Geometry check sheet. Reference: the model listing, model coordinates, mm. Face numbers are marked on the shaded views. A direction names the side the tool comes from. Round coordinates to 2 decimals unless told otherwise and drop trailing zeros. Order: outer loops, then holes, each group sorted by start corner. A loop starts at its lowest first (then second) coordinate and runs counter-clockwise, first axis right, second up.
(1) Cross-section at A-A on y = 0. Enter the section's corners in (x, z) (3 decimals), and give its area (3 significant figures).
(2) Thickness scan on L1, parallel to Z at x = 5, y = 0; L2, parallel to X at y = -6.5, z = 0.5; L3, parallel to X at y = 1.5, z = 3.75. Record the ranges inside material, lowest first.
(3) Gauge pin test, flat ends, axial feed: P1, Ø4, axis at x = 19, z = -4, coming from the +Y side; P2, Ø1.5, axis at x = 13, z = 1.5, coming from the -Y side; P3, Ø1, axis at x = 4, z = -4, coming from the +Y side. Record the tip position at first contact, or that the pin passes through.
(4) Cross-section at B-B on z = 0. Enter the section's corners in (x, y) (3 decimals).
(5) Set-up check for the marked faces 1 and 2: record each of +Z, -Z, +X, -X, +Y, -Y from which the full face is reachable in a straight line by a thin tool's end or side.
(6) Cross-section at C-C on x = 10.5. Enter the section's corners in (y, z), and give its area (3 significant figures).
from build123d import *

# Parameters (mm, degrees)
SKETCH_2_OUTSIDE_W  = 23.47
SKETCH_2_OUTSIDE_H  = 23.47
CUT_EXTRUDE_1_DEPTH = 30.3


with BuildPart() as part:
    # Эскиз1 → Повернуть1 (revolve)
    with BuildSketch(Plane.XY):
        Polygon((-5.3, 0), (-5.3, 6.175), (-5.052146997, 7.1), (0, 7.1), (0, 4), (24.2, 4), (25, 3.2), (25, 0), align=None)
    revolve(axis=Axis((-1000, 0, 0), (1, 0, 0)))

    # Эскиз2 outside → Вырез-Вытянуть1 (cut)
    with BuildSketch(Plane.ZY.offset(5.3)):
        Rectangle(SKETCH_2_OUTSIDE_W, SKETCH_2_OUTSIDE_H)
        Polygon((0, 7.505553499), (-6.5, 3.75277675), (-6.5, -3.75277675), (0, -7.505553499), (6.5, -3.75277675), (6.5, 3.75277675), align=None, mode=Mode.SUBTRACT)
    extrude(amount=-CUT_EXTRUDE_1_DEPTH, mode=Mode.SUBTRACT)


solid = part.part
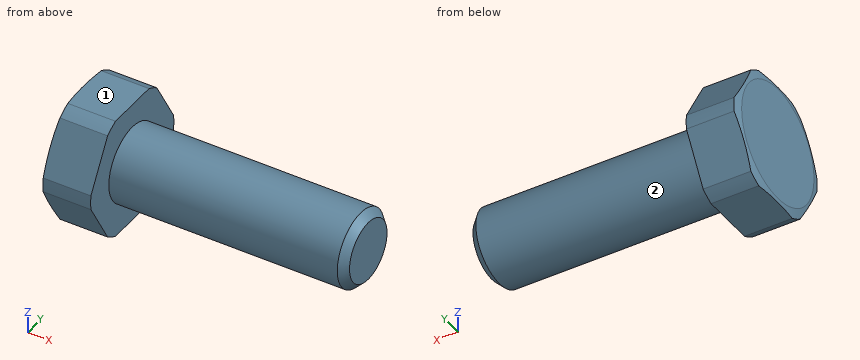
Found:
1. outline: (-5.3, -6.175) - (-5.213, -6.5) - (0, -6.5) - (0, -4) - (24.2, -4) - (25, -3.2) - (25, 3.2) - (24.2, 4) - (0, 4) - (0, 6.5) - (-5.213, 6.5) - (-5.3, 6.175) - close
1. area: 268 mm2
2. L1: z = -4 to 4
2. L2: x = -5.21 to 0
2. L3: x = -5.3 to 0
3. P1: stops at y = 3.46
3. P2: stops at y = -3.93
3. P3: stops at y = 1.94
4. outline: (-5.3, -6.175) - (-5.052, -7.1) - (0, -7.1) - (0, -4) - (24.2, -4) - (25, -3.2) - (25, 3.2) - (24.2, 4) - (0, 4) - (0, 7.1) - (-5.052, 7.1) - (-5.3, 6.175) - close
5. face 1: +Z, +X, -X, +Y, -Y
5. face 2: +X
6. outline: circle Ø8 at (0, 0)
6. area: 50.3 mm2
